```python
from build123d import *

# Parameters (mm, degrees)
BOSS_EXTRUDE1_DEPTH = 10
CUT_EXTRUDE39_DEPTH = 10


with BuildPart() as part:
    # Sketch1 → Boss-Extrude1 (new body)
    with BuildSketch(Plane.XY):
        with BuildLine():
            Line((-50, 60), (50, 60))
            ThreePointArc((50, 60), (57.071067812, 57.071067812), (60, 50))
            Line((60, 50), (60, -50))
            ThreePointArc((60, -50), (57.071067812, -57.071067812), (50, -60))
            Line((50, -60), (-50, -60))
            ThreePointArc((-50, -60), (-57.071067812, -57.071067812), (-60, -50))
            Line((-60, -50), (-60, 50))
            ThreePointArc((-60, 50), (-57.071067812, 57.071067812), (-50, 60))
        make_face()
    extrude(amount=BOSS_EXTRUDE1_DEPTH)

    # Sketch2 → Cut-Extrude39 (cut)
    with BuildSketch(Plane.XY.offset(10)):
        Polygon((-28.58974359, 50), (31.666666667, 50), (-4.150641026, -32.051282051), (29.102564103, -32.051282051), (29.102564103, -50), (-31.153846154, -50), (4.68349359, 32.051282051), (-28.58974359, 32.051282051), align=None)
    extrude(amount=-CUT_EXTRUDE39_DEPTH, mode=Mode.SUBTRACT)


solid = part.part
```
Geometry: final body of the model. Coordinates: model frame, mm. A direction names the side the tool comes from. Coordinates: 2 decimals unless noted, no trailing zeros. Order: outer loops, then holes, each group sorted by start corner. A loop starts at its lowest first (then second) coordinate and runs counter-clockwise, first axis right, second up. Notation, with made-up numbers: (87, 72) -> (129, 72) arc R33 cw to (129, 106) -> close; hole circle Ø6 at (38.25, 52.5). An arc over 180 degrees is marked (long way). Use CSV: the item, a comma, the result in double quotes.
1) Section D-D on y = -35. Output: boundary loops of the cut face in (x, z).
Findings:
outline,"(-60, 0) -> (-24.6, 0) -> (-24.6, 10) -> (-60, 10) -> close; (29.1, 0) -> (60, 0) -> (60, 10) -> (29.1, 10) -> close"
2) Line query: line 1 (Y direction, x = 20, z = 6); line 2 (Y direction, x = -2, z = 6); line 3 (Y direction, x = -15.5, z = 4.5). Output: solid intervals per line, ascending.
Findings:
line 1,"y = -60 to -50, -32.05 to 23.27, 50 to 60"
line 2,"y = -60 to -50, -32.05 to -27.12, 16.75 to 32.05, 50 to 60"
line 3,"y = -60 to -50, -14.16 to 32.05, 50 to 60"
3) Pin query (flat end, axial travel): pin 1 Ø10 at (x, y) = (41, -20) entering from -Z. Return the tip coordinate at first contact, or that it passes through.
Findings:
pin 1,"stops at z = 0"
4) Section C-C on x = 1. Output: boundary loops of the cut face in (y, z), then the cut area to 3 significant figures.
Findings:
outline,"(-60, 0) -> (-50, 0) -> (-50, 10) -> (-60, 10) -> close; (-32.05, 0) -> (-20.25, 0) -> (-20.25, 10) -> (-32.05, 10) -> close; (23.62, 0) -> (32.05, 0) -> (32.05, 10) -> (23.62, 10) -> close; (50, 0) -> (60, 0) -> (60, 10) -> (50, 10) -> close"
area,"402 mm^2"
5) Section A-A on y = -14. Output: boundary loops of the cut face in (x, z).
Findings:
outline,"(-60, 0) -> (-15.43, 0) -> (-15.43, 10) -> (-60, 10) -> close; (3.73, 0) -> (60, 0) -> (60, 10) -> (3.73, 10) -> close"
6) Section B-B on z = 7.75. Output: boundary loops of the cut face in (x, y), then the cut area to 3 significant figures.
Findings:
outline,"(-60, -50) arc R10 ccw to (-50, -60) -> (50, -60) arc R10 ccw to (60, -50) -> (60, 50) arc R10 ccw to (50, 60) -> (-50, 60) arc R10 ccw to (-60, 50) -> close; hole (-31.15, -50) -> (29.1, -50) -> (29.1, -32.05) -> (-4.15, -32.05) -> (31.67, 50) -> (-28.59, 50) -> (-28.59, 32.05) -> (4.68, 32.05) -> close"
area,"11,100 mm^2"
7) Mould query, pull axis Y, two halves, no side actions, for faces 3 (the flat face through (-1, 60, 5)), 4 (the flat face through (-28.59, 41, 5)), 5 (the flat face through (14, 1, 10)). Classes: +Y half, -Y half, draft (parallel to the pull), parting line (faces both ways), or undercut.
Findings:
face 3,"+Y half"
face 4,"undercut"
face 5,"draft"
8) Access query for faces 1 (the flat face through (-60, -1, 5)), 2 (the flat face through (29.103, -41, 5)). Directions: +Z, -Z, +X, -X, +Y, -Y. A direction counts if a zero-diameter tool reaches every point of the face in a straight line with its end or side. Return the directions, or none.
Findings:
face 1,"+Z, -Z, -X, +Y, -Y"
face 2,"+Z, -Z"
